```python
from build123d import *

# Parameters (mm, degrees)
SKETCH_2_W          = 24
SKETCH_2_H          = 61.5
SKETCH_2_R          = 1.75
EXTRUDE_1_DEPTH     = 2
SKETCH_3_W          = 17
SKETCH_3_H          = 30
EXTRUDE_2_DEPTH     = 16.75
SKETCH_4_R          = 2.25
CUT_EXTRUDE_1_DEPTH = 69.628073702
EXTRUDE_3_DEPTH     = 1.5
EXTRUDE_START       = -2
SKETCH_6_R          = 1.75
EXTRUDE_4_DEPTH     = 2
SKETCH_7_R          = 1.75
CUT_EXTRUDE_2_DEPTH = 69.108828356


with BuildPart() as part:
    # 草图2 → 凸台-拉伸1 (new body)
    with BuildSketch(Plane.XY):
        with Locations((12, 30.75)):
            Rectangle(SKETCH_2_W, SKETCH_2_H)
        with Locations((5, 56.5)):
            Circle(SKETCH_2_R, mode=Mode.SUBTRACT)
        with Locations((19, 56.5)):
            Circle(SKETCH_2_R, mode=Mode.SUBTRACT)
        with Locations((5, 5)):
            Circle(SKETCH_2_R, mode=Mode.SUBTRACT)
        with Locations((19, 5)):
            Circle(SKETCH_2_R, mode=Mode.SUBTRACT)
    extrude(amount=EXTRUDE_1_DEPTH)

    # 草图3 → 凸台-拉伸2 (add)
    with BuildSketch(Plane.XY.offset(2)):
        with Locations((12, 30.75)):
            Rectangle(SKETCH_3_W, SKETCH_3_H)
    extrude(amount=EXTRUDE_2_DEPTH)

    # 草图4 → 切除-拉伸1 (cut, through all)
    with BuildSketch(Plane(origin=(24, 0, 0), x_dir=(0, 0, -1), z_dir=(1, 0, 0))):
        with Locations(Location((-13.75, 23.25, 0), (0, 0, 270))):
            Circle(SKETCH_4_R)
        with Locations(Location((-13.75, 38.25, 0), (0, 0, 270))):
            Circle(SKETCH_4_R)
    extrude(amount=-CUT_EXTRUDE_1_DEPTH, mode=Mode.SUBTRACT)

    # 草图5 → 凸台-拉伸3 (add, symmetric)
    with BuildSketch(Plane(origin=(12, 0, 0), x_dir=(0, 0, -1), z_dir=(1, 0, 0))):
        Polygon((-2, 56.142304845), (-2, 45.75), (-8, 45.75), align=None)
        Polygon((-2, 15.75), (-2, 5.357695155), (-8, 15.75), align=None)
    extrude(amount=EXTRUDE_3_DEPTH, both=True)

    # 草图6 → 凸台-拉伸4 (add)
    with BuildSketch(Plane.XY.offset(2).offset(EXTRUDE_START)):
        with Locations((5, 56.5)):
            Circle(SKETCH_6_R)
        with Locations((19, 56.5)):
            Circle(SKETCH_6_R)
        with Locations((19, 5)):
            Circle(SKETCH_6_R)
        with Locations((5, 5)):
            Circle(SKETCH_6_R)
    extrude(amount=EXTRUDE_4_DEPTH)

    # 草图7 → 切除-拉伸2 (cut, through all)
    with BuildSketch(Plane.XY.offset(2)):
        with Locations((4.25, 57.25)):
            Circle(SKETCH_7_R)
        with Locations((19.75, 57.25)):
            Circle(SKETCH_7_R)
        with Locations((4.25, 4.25)):
            Circle(SKETCH_7_R)
        with Locations((19.75, 4.25)):
            Circle(SKETCH_7_R)
    extrude(amount=-CUT_EXTRUDE_2_DEPTH, mode=Mode.SUBTRACT)


solid = part.part
```
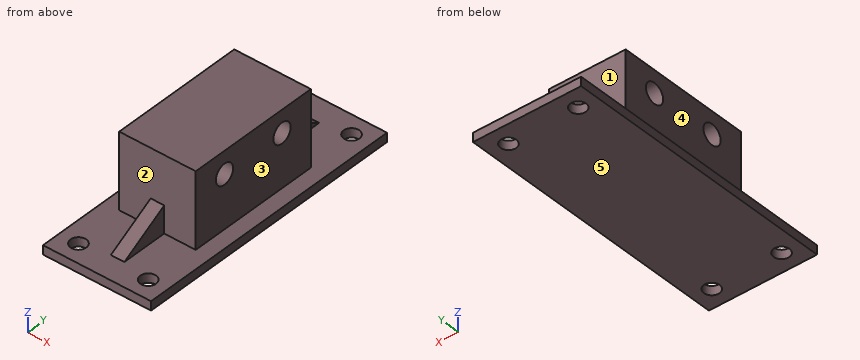
Build history of the part. All positions in model axes, mm. Face numbers are marked on the shaded views. A direction names the side the tool comes from. Round coordinates to 2 decimals unless told otherwise and drop trailing zeros. Write each loop counter-clockwise with the first axis right and the second up, starting at its lowest first coordinate (ties: lowest second). Pieces come first, ordered by that corner, then holes.
1) Drill centre lines: probe 1 along Y at (x, z) = (18.5, 13.75); probe 2 along Y at (x, z) = (4.25, 0.85); probe 3 along Z at (x, y) = (11, 23.25). Where is each one in solid material? Low to high.
2) 3-axis set-ups, long thin cutter, end or side, ignore diameter. For the marked faces 1, 2, 3, 4 and 5: which of +Z, -Z, +X, -X, +Y, -Y reach the whole face in a straight line?
3) Band-saw the part on C-C, the plane z = 13.75. List the corners of the cut face in (x, y), and give its area (3 significant figures).
4) Band-saw the part on B-B, the plane y = 38.25. List the corners of the cut face in (x, z).
5) Band-saw the part on D-D, the plane y = 30. List the corners of the cut face in (x, z).
6) Pin check, flat tips, straight feed: pin 1 (5 mm diameter, centred on y = 11, z = 6.5, fed in from +X); pin 2 (1.5 mm diameter, centred on y = 44.5, z = 6.5, fed in from -X); pin 3 (10 mm diameter, centred on x = 4, z = 16, fed in from +Y). Stop position of each tip, or through.
7) Band-saw the part on A-A, the plane x = 19.75. List the corners of the cut face in (y, z), and give its area (3 significant figures).
Ans:
1. probe 1: y = 15.75 to 21, 25.5 to 36, 40.5 to 45.75
1. probe 2: y = 0 to 2.5, 6 to 55.5, 59 to 61.5
1. probe 3: z = 0 to 11.5, 16 to 18.75
2. face 1: +Z, +Y
2. face 2: +Z, -Y
2. face 3: +Z, +X, +Y, -Y
2. face 4: +Z, -X, +Y, -Y
2. face 5: -Z, +X, -X, +Y, -Y
3. outline: (3.5, 15.75) - (20.5, 15.75) - (20.5, 21) - (3.5, 21) - close; (3.5, 25.5) - (20.5, 25.5) - (20.5, 36) - (3.5, 36) - close; (3.5, 40.5) - (20.5, 40.5) - (20.5, 45.75) - (3.5, 45.75) - close
3. area: 357 mm2
4. outline: (0, 0) - (24, 0) - (24, 2) - (20.5, 2) - (20.5, 11.5) - (3.5, 11.5) - (3.5, 2) - (0, 2) - close; (3.5, 16) - (20.5, 16) - (20.5, 18.75) - (3.5, 18.75) - close
5. outline: (0, 0) - (24, 0) - (24, 2) - (20.5, 2) - (20.5, 18.75) - (3.5, 18.75) - (3.5, 2) - (0, 2) - close
6. pin 1: stops at x = 13.5
6. pin 2: stops at x = 3.5
6. pin 3: stops at y = 45.75
7. outline: (0, 0) - (2.5, 0) - (2.5, 2) - (0, 2) - close; (6, 0) - (55.5, 0) - (55.5, 2) - (45.75, 2) - (45.75, 18.75) - (15.75, 18.75) - (15.75, 2) - (6, 2) - close; (59, 0) - (61.5, 0) - (61.5, 2) - (59, 2) - close; hole circle Ø4.5 at (23.25, 13.75); hole circle Ø4.5 at (38.25, 13.75)
7. area: 580 mm2
